```python
from build123d import *

# Parameters (mm, degrees)
F0_W     = 900
F0_H     = 100
F1_DEPTH = 45
F3_DEPTH = 130.1


with BuildPart() as f1:
    # F0 (on Top) → F1 (new body)
    with BuildSketch(Plane.XY):
        Rectangle(F0_W, F0_H)
    extrude(amount=F1_DEPTH)

    # F2 (on face) → F3 (cut)
    with BuildSketch(Plane.XY.offset(45)):
        with BuildLine():
            ThreePointArc((-410, 0), (-405, -5), (-400, 0))
            ThreePointArc((-400, 0), (-405, 5), (-410, 0))
        make_face()
    extrude(amount=-F3_DEPTH, mode=Mode.SUBTRACT)


solid = f1.part
```
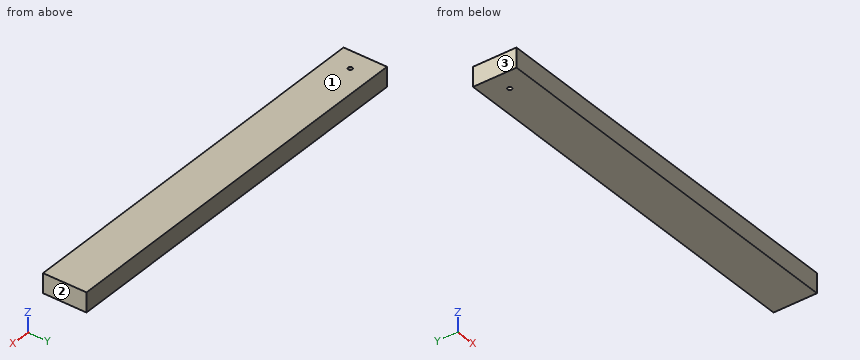
Source: CAD feature listing. Evaluate the final solid. Frame: model axes, mm. Face numbers are marked on the shaded views. Give positions to 0.01 mm unless a question says otherwise; leave off trailing zeros. One line per item, written item: value. Start each with the question number.
Q1. Draft query along X for the marked faces 1, 2 and 3. Return one class per face: +X half, -X half, draft (parallel to the pull), parting line (faces both ways), or undercut.
Q2. Material intervals for probe 1 along Y at (x, z) = (-405, 28); probe 2 along X at (y, z) = (-4.5, 13.5), sorted ascending. Write a range as from..to.
Q3. First-contact query: pin 1 Ø9 at (x, y) = (-405, 0) entering from +Z. Flat tip, straight axial feed; report the tip coordinate or a pass-through.
Answer:
1. face 1: draft
1. face 2: +X half
1. face 3: -X half
2. probe 1: y = -50..-5, 5..50
2. probe 2: x = -450..-407.18, -402.82..450
3. pin 1: passes through
